Drawing for the job (mm, zero at the part's lowest x, y, z). A direction names the side the tool comes from. Give positions to 0.01 mm unless a question says otherwise; leave off trailing zeros. Loops run counter-clockwise (first coordinate to the right, second up) from the corner with the lowest first, then second, coordinate; pieces in that order, holes last. Notation, with made-up numbers: (43, 5.5) - (100, 5.5) arc R25 cw to (100, 39.5) - close; hole circle Ø11 at (78, -30). An arc over 180 degrees is marked (long way). Return JSON: item names as keys, results as strings. Group by question number.
1) Drop flat-ended pins along their axis: pin 1 (1 mm diameter, centred on x = 19.5, z = 15.5, fed in from +Y); pin 2 (16.5 mm diameter, centred on x = 14.875, y = 13.95, fed in from -Z); pin 3 (8 mm diameter, centred on x = 16.5, y = 13.5, fed in from +Z); pin 4 (10 mm diameter, centred on x = 13, z = 17, fed in from -Y). Give the stop position or say it passes through.
2) Slice it at B-B (x = 20.5). List the corners of the cut face in (y, z), and give its area (3 significant figures).
3) Slice it at A-A (y = 13.95). List the corners of the cut face in (x, z).
4) 3-axis set-ups, long thin cutter, end or side, ignore diameter. For the marked faces 5, 6 and 7: which of +Z, -Z, +X, -X, +Y, -Y reach the whole face in a straight line?
5) Slice it at C-C (z = 11). List the corners of the cut face in (x, y) (3 decimals).
6) Drill centre lines: probe 1 along Y at (x, z) = (23.5, 12.5); probe 2 along X at (y, z) = (18.25, 2); probe 3 along X at (y, z) = (12, 18). Where is each one in solid material? Low to high. Write a range as from..to.
7) Mould opens along X. For the marked faces 1, 2, 3 and 4 say: released by +X, released by -X, zero draft, split by the parting line, or undercut.
8) Slice it at D-D (x = 26.75). List the corners of the cut face in (y, z), and give its area (3 significant figures).
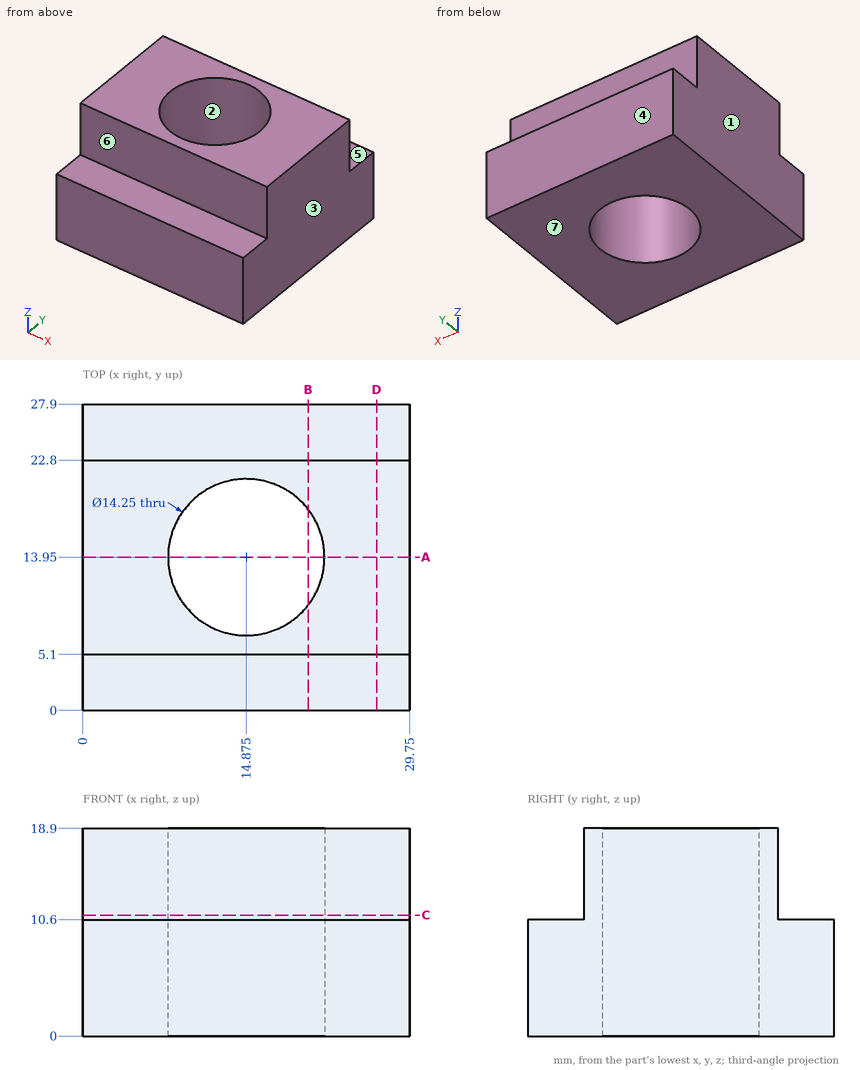
Results:
{
 "1": {"pin 1": "y = 22.8", "pin 2": "z = 0", "pin 3": "through", "pin 4": "y = 5.1"},
 "2": {"outline": "(0, 0) - (9.58, 0) - (9.58, 18.9) - (5.1, 18.9) - (5.1, 10.6) - (0, 10.6) - close; (18.32, 0) - (27.9, 0) - (27.9, 10.6) - (22.8, 10.6) - (22.8, 18.9) - (18.32, 18.9) - close", "area": "277 mm2"},
 "3": {"outline": "(0, 0) - (7.75, 0) - (7.75, 18.9) - (0, 18.9) - close; (22, 0) - (29.75, 0) - (29.75, 18.9) - (22, 18.9) - close"},
 "4": {"face 5": "+Z, +X, -X, +Y", "face 6": "+Z, +X, -X, -Y", "face 7": "-Z, +X, -X, +Y, -Y"},
 "5": {"outline": "(0, 5.1) - (29.75, 5.1) - (29.75, 22.8) - (0, 22.8) - close; hole circle Ø14.25 at (14.875, 13.95)"},
 "6": {"probe 1": "5.1..22.8", "probe 2": "0..9.19, 20.56..29.75", "probe 3": "0..8.02, 21.73..29.75"},
 "7": {"face 1": "released by -X", "face 2": "undercut", "face 3": "released by +X", "face 4": "zero draft"},
 "8": {"outline": "(0, 0) - (27.9, 0) - (27.9, 10.6) - (22.8, 10.6) - (22.8, 18.9) - (5.1, 18.9) - (5.1, 10.6) - (0, 10.6) - close", "area": "443 mm2"}
}
